For this review, take the finished solid that the model builds, in its own axes (mm). Face numbers are marked on the shaded views. A direction names the side the tool comes from. Round coordinates to 2 decimals unless told otherwise and drop trailing zeros. Loops run counter-clockwise (first coordinate to the right, second up) from the corner with the lowest first, then second, coordinate; pieces in that order, holes last.
1. Clearance check with flat-ended pins moving along their axes: pin 1 Ø3 at (x, y) = (1, -3) entering from +Z; pin 2 Ø2 at (x, y) = (4, -8) entering from -Z. State where each tip first meets the part, or that it passes through.
2. Tool access review of the marked faces 1 and 2: name each direction out of +Z, -Z, +X, -X, +Y, -Y from which nothing blocks a thin tool from reaching the whole face with its end or side.
3. Draft analysis for pull direction Y (two halves, no side actions). For the marked faces 3 and 4, state which applies: released by +Y, released by -Y, zero draft, split by the parting line, or undercut.
4. Consider section B-B on y = -5.5. State the section outline as (x, z) points.
5. Consider section C-C on x = 1. State the section outline as (y, z) points, then the cut area to 3 significant figures.
6. Consider section A-A on z = 0.75. State the section outline as (x, y) points, then the cut area to 3 significant figures.
7. To check wall thickness, follow line 1 along Y through (x, z) = (2.75, 0.4); line 2 along Y through (x, z) = (-3.25, 0.75); line 3 along X through (y, z) = (6.75, 0.8). State the ranges of each line that lie inside material, in increasing order.
8. Consider section D-D on x = -4.75. State the section outline as (y, z) points.
Autodesk Inventor part; units mm, degrees
ref_plane "YZ Plane" through (0, 0, 0) normal (1, 0, 0) x (0, 1, 0)
ref_plane "XZ Plane" through (0, 0, 0) normal (0, 1, 0) x (-1, 0, 0)
ref_plane "XY Plane" through (0, 0, 0) normal (0, 0, 1) x (1, 0, 0)
sketch "Sketch1" plane through (0, 0, 0) normal (0, 0, 1) x (1, 0, 0)
  line L0 (-7, 12.5) -> (7, 12.5)
  line L1 (7, 12.5) -> (7, -12.5)
  line L2 (7, -12.5) -> (-7, -12.5)
  line L3 (-7, -12.5) -> (-7, 12.5)
  point P0 (0, 0)
  point P1 (7, 0)
  point P2 (0, 12.5)
  dimension "d0" = 14
  dimension "d1" = 25
extrude "Extrusion1" add sketch "Sketch1" along normal blind 1
sketch "Sketch2" plane through (0, 0, 1) normal (0, 0, 1) x (1, 0, 0)
  line L0 (-5.5, 11.5) -> (5.5, 11.5)
  line L1 (5.5, 11.5) -> (5.5, 0.5)
  line L2 (5.5, 0.5) -> (-5.5, 0.5)
  line L3 (-5.5, 0.5) -> (-5.5, 11.5)
  line L4 (7, 12.5) -> (-7, 12.5)
  point P0 (0, 0)
  point P1 (0, 11.5)
  dimension "d4" = 11
  dimension "d5" = 11
  dimension "d6" = 1
extrude "Extrusion2" cut sketch "Sketch2" against normal blind 0.4
sketch "Sketch3" plane through (0, 0, 0.6) normal (0, 0, 1) x (1, 0, 0)
  line L0 (5.5, 0.5) -> (-5.5, 0.5)
  line L1 (5.5, 11.5) -> (5.5, 0.5)
  line L2 (-5.5, 11.5) -> (5.5, 11.5)
  line L3 (-5.5, 0.5) -> (-5.5, 11.5)
  line L4 (4, 10) -> (4, 2)
  line L5 (4, 2) -> (-4, 2)
  line L6 (-4, 2) -> (-4, 10)
  line L7 (-4, 10) -> (4, 10)
  point P0 (0, 0)
  dimension "d9" = 1.5
extrude "Extrusion3" cut sketch "Sketch3" against normal through all contours L4 L5 L6 L7
mirror "Mirror1" about plane through (0, 0, 0) normal (0, 1, 0) of "Extrusion3", "Extrusion2"
fillet "Fillet1" radius 2 4 edges at (7, 12.5, 0.5) (7, -12.5, 0.5) (-7, -12.5, 0.5) (-7, 12.5, 0.5)
fillet "Fillet2" radius 0.5 8 edges at (-4, 2, 0.3) (-4, 10, 0.3) (4, 10, 0.3) (4, 2, 0.3) (4, -2, 0.3) (-4, -2, 0.3) (-4, -10, 0.3) (4, -10, 0.3)
fillet "Fillet3" radius 0.5 8 edges at (-5.5, 11.5, 0.8) (5.5, 11.5, 0.8) (5.5, 0.5, 0.8) (-5.5, 0.5, 0.8) (-5.5, -0.5, 0.8) (5.5, -0.5, 0.8) (5.5, -11.5, 0.8) (-5.5, -11.5, 0.8)
properties part number "SampleTray" material "UHMW, White"
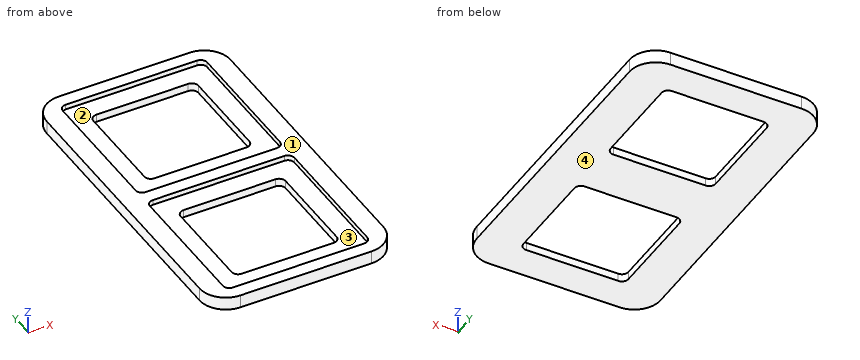
Resolved:
1. pin 1: stops at z = 0.6
1. pin 2: stops at z = 0
2. face 1: +Z, +X, -X, +Y, -Y
2. face 2: +Z
3. face 3: undercut
3. face 4: zero draft
4. outline: (-7, 0) - (-4, 0) - (-4, 0.6) - (-5.5, 0.6) - (-5.5, 1) - (-7, 1) - close; (4, 0) - (7, 0) - (7, 1) - (5.5, 1) - (5.5, 0.6) - (4, 0.6) - close
5. outline: (-12.5, 0) - (-10, 0) - (-10, 0.6) - (-11.5, 0.6) - (-11.5, 1) - (-12.5, 1) - close; (-2, 0) - (2, 0) - (2, 0.6) - (0.5, 0.6) - (0.5, 1) - (-0.5, 1) - (-0.5, 0.6) - (-2, 0.6) - close; (10, 0) - (12.5, 0) - (12.5, 1) - (11.5, 1) - (11.5, 0.6) - (10, 0.6) - close
5. area: 6.60 mm2
6. outline: (-7, -10.5) arc R2 ccw to (-5, -12.5) - (5, -12.5) arc R2 ccw to (7, -10.5) - (7, 10.5) arc R2 ccw to (5, 12.5) - (-5, 12.5) arc R2 ccw to (-7, 10.5) - close; hole (-5.5, -11) arc R0.5 ccw to (-5, -11.5) - (5, -11.5) arc R0.5 ccw to (5.5, -11) - (5.5, -1) arc R0.5 ccw to (5, -0.5) - (-5, -0.5) arc R0.5 ccw to (-5.5, -1) - close; hole (-5.5, 1) arc R0.5 ccw to (-5, 0.5) - (5, 0.5) arc R0.5 ccw to (5.5, 1) - (5.5, 11) arc R0.5 ccw to (5, 11.5) - (-5, 11.5) arc R0.5 ccw to (-5.5, 11) - close
6. area: 105 mm2
7. line 1: y = -12.5 to -10, -2 to 2, 10 to 12.5
7. line 2: y = -12.5 to -11.5, -0.5 to 0.5, 11.5 to 12.5
7. line 3: x = -7 to -5.5, 5.5 to 7
8. outline: (-12.5, 0) - (12.5, 0) - (12.5, 1) - (11.5, 1) - (11.5, 0.6) - (0.5, 0.6) - (0.5, 1) - (-0.5, 1) - (-0.5, 0.6) - (-11.5, 0.6) - (-11.5, 1) - (-12.5, 1) - close
